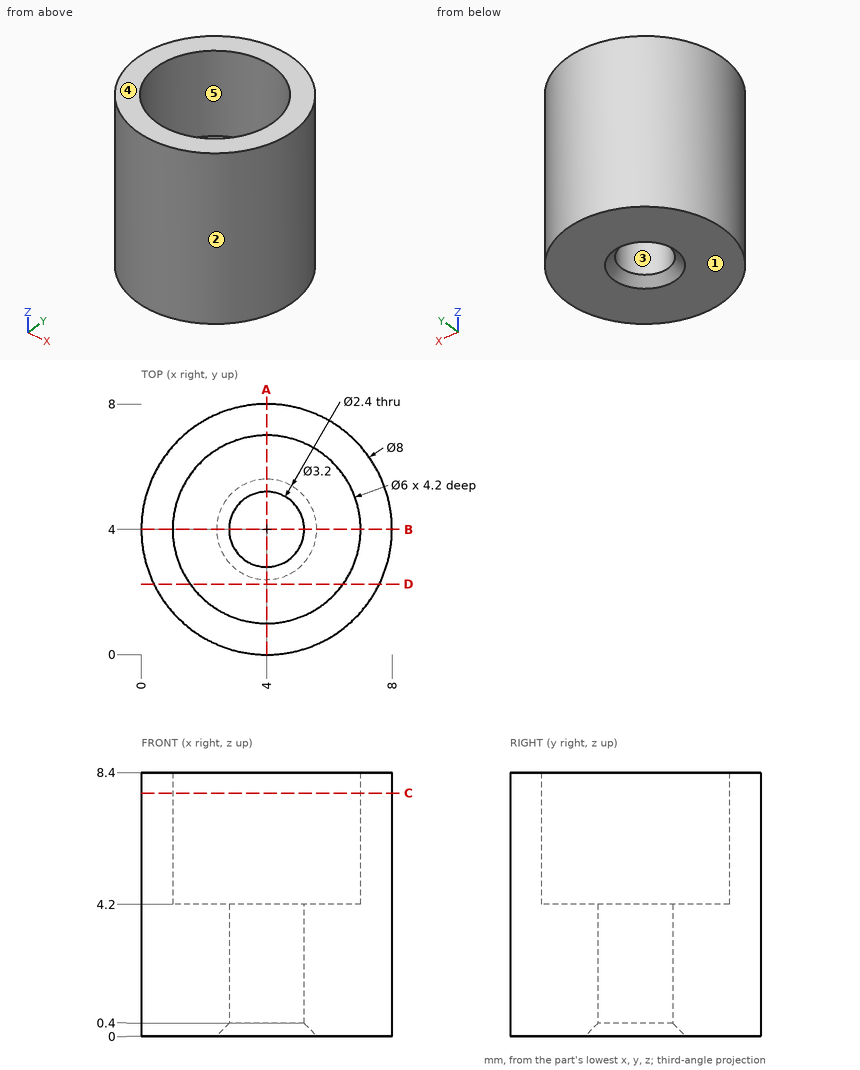
Job drawing, mm, ordinate dimensions from the low corner. One solid piece. A direction names the side the tool comes from. Give positions to 0.01 mm unless a question says otherwise; leave off trailing zeros. Loops run counter-clockwise (first coordinate to the right, second up) from the corner with the lowest first, then second, coordinate; pieces in that order, holes last. Notation, with made-up numbers: M 59.5,42 L 77.5,42 A28 ccw 77.5,75 Z; hole C -11.75,-17.75 d9. An arc over 180 degrees is marked long. Answer in a Markdown table with one row per item. Add a question column.
Item 1: Drop flat-ended pins along their axis: P1, Ø4, axis at x = 7, y = 2.5, coming from the -Z side; P2, Ø3, axis at x = 2, z = 4.5, coming from the -Y side; P3, Ø1.5, axis at y = 6.5, z = 7, coming from the -X side; P4, Ø1.4, axis at x = 4, y = 4, coming from the +Z side. Give the stop position or say it passes through.
Item 2: Band-saw the part on D-D on y = 2.25. Give the cut face in (x, z).
Item 3: Tool access for the marked faces 4 and 5: list every direction of +Z, -Z, +X, -X, +Y, -Y with a clear straight run to the whole face (end or side of a thin tool).
Item 4: Band-saw the part on A-A on x = 4. Give the cut face in (y, z), then the cut area to 3 significant figures.
Item 5: Mould opens along Y. For the marked faces 1, 2 and 3 say: +Y half, -Y half, draft (parallel to the pull), parting line (faces both ways), or undercut.
Item 6: Band-saw the part on C-C on z = 7.75. Give the cut face in (x, y).
Item 7: Probe probe 1 along Y at (x, z) = (4, 2.35); probe 2 along Z at (x, y) = (3.25, 2.5); probe 3 along Y at (x, z) = (4, 7.2). List the from-to ranges inside material, lowest first.
Reply:
| question | item | result |
|---|---|---|
| 1 | P1 | stops at z = 0 |
| 1 | P2 | stops at y = 0.03 |
| 1 | P3 | stops at x = 0.4 |
| 1 | P4 | passes through |
| 2 | outline | M 0.4,0 L 7.6,0 L 7.6,8.4 L 6.44,8.4 L 6.44,4.2 L 1.56,4.2 L 1.56,8.4 L 0.4,8.4 Z |
| 3 | face 4 | +Z, +X, -X, +Y, -Y |
| 3 | face 5 | +Z |
| 4 | outline | M 0,0 L 2.4,0 L 2.8,0.4 L 2.8,4.2 L 1,4.2 L 1,8.4 L 0,8.4 Z; M 5.2,0.4 L 5.6,0 L 8,0 L 8,8.4 L 7,8.4 L 7,4.2 L 5.2,4.2 Z |
| 4 | area | 31.8 mm^2 |
| 5 | face 1 | draft |
| 5 | face 2 | parting line |
| 5 | face 3 | undercut |
| 6 | outline | C 4,4 d8; hole C 4,4 d6 |
| 7 | probe 1 | y = 0 to 2.8, 5.2 to 8 |
| 7 | probe 2 | z = 0 to 4.2 |
| 7 | probe 3 | y = 0 to 1, 7 to 8 |
